Verification items for the finished model (mm, model axes). Face numbers are marked on the shaded views. A direction names the side the tool comes from. Give positions to 0.01 mm unless a question says otherwise; leave off trailing zeros. Loops run counter-clockwise (first coordinate to the right, second up) from the corner with the lowest first, then second, coordinate; pieces in that order, holes last. Notation, with made-up numbers: M -26,-5.75 L 27,-5.75 A22 ccw 27,4.25 Z; hole C 22,46 d5. An arc over 180 degrees is marked long. Put each result on its own line as item: value. Start each with the question number.
from build123d import *

# Parameters (mm, degrees)
F1_DEPTH = 24.85502


# Not quite as in the source:
# - ends of sketch curves that miss each other by under 0.0002 mm in the source are joined


with BuildPart() as f1:
    # F0 (on Top) → F1 (new body)
    with BuildSketch(Plane.XY):
        with BuildLine():
            Line((31.75, -31.7133048595), (44.45, -31.7133048595))
            ThreePointArc((44.45, -31.7133048595), (42.0664322772, -17.3530202013), (35.171359934, -4.5328350256))
            ThreePointArc((35.171359934, -4.5328350256), (33.2360090694, -2.1977123508), (31.1459274206, 0))
            Line((31.1459274206, 0), (1.526038953, 0))
            ThreePointArc((1.526038953, 0), (22.9838447258, -9.8088445461), (31.75, -31.7133048595))
        make_face()
        with BuildLine():
            Line((44.45, -40.8569961303), (44.45, -31.7133048595))
            ThreePointArc((44.45, -31.7133048595), (44.2101126583, -36.3250766164), (43.4930398768, -40.8870708405))
            ThreePointArc((43.4930398768, -40.8870708405), (43.9712837047, -40.8645166634), (44.45, -40.8569961303))
        make_face()
        with BuildLine():
            ThreePointArc((43.4930398768, -40.8870708405), (44.2101126583, -36.3250766164), (44.45, -31.7133048595))
            Line((44.45, -31.7133048595), (31.75, -31.7133048595))
            ThreePointArc((31.75, -31.7133048595), (22.4506403027, -54.1639451622), (0, -63.4633048595))
            Line((0, -63.4633048595), (31.1085197333, -63.4633048595))
            ThreePointArc((31.1085197333, -63.4633048595), (31.0883782789, -48.7672850184), (43.4930398768, -40.8870708405))
        make_face()
        with BuildLine():
            ThreePointArc((35.171359934, -4.5328350256), (42.0664322772, -17.3530202013), (44.45, -31.7133048595))
            Line((44.45, -31.7133048595), (44.45, -4.5328350256))
            Line((44.45, -4.5328350256), (35.171359934, -4.5328350256))
        make_face()
        with BuildLine():
            Line((44.45, -4.5328350256), (44.45, -31.7133048595))
            Line((44.45, -31.7133048595), (44.45, -40.8569961303))
            ThreePointArc((44.45, -40.8569961303), (52.1958071052, -42.9722076639), (57.7914802832, -48.730687431))
            ThreePointArc((57.7914802832, -48.730687431), (63.7666518684, -28.0228983697), (84.4744408875, -33.9980701011))
            ThreePointArc((84.4744408875, -33.9980701011), (90.4496122897, -13.290280973), (111.1574013682, -19.2654525473))
            ThreePointArc((111.1574013682, -19.2654525473), (109.2588815999, -11.8991437909), (111.1574013333, -4.5328350256))
            Line((111.1574013333, -4.5328350256), (44.45, -4.5328350256))
        make_face()
        with BuildLine():
            ThreePointArc((44.45, -40.8569961303), (43.9712837047, -40.8645166634), (43.4930398768, -40.8870708405))
            ThreePointArc((43.4930398768, -40.8870708405), (38.9713966864, -53.0916289358), (31.1085197333, -63.4633048595))
            Line((31.1085197333, -63.4633048595), (44.45, -56.0969961303))
            Line((44.45, -56.0969961303), (44.45, -40.8569961303))
        make_face()
        with BuildLine():
            ThreePointArc((31.1085197333, -63.4633048595), (38.9713966864, -53.0916289358), (43.4930398768, -40.8870708405))
            ThreePointArc((43.4930398768, -40.8870708405), (31.0883782789, -48.7672850184), (31.1085197333, -63.4633048595))
        make_face()
        with BuildLine():
            ThreePointArc((57.7914802832, -48.730687431), (52.1958071052, -42.9722076639), (44.45, -40.8569961303))
            Line((44.45, -40.8569961303), (44.45, -56.0969961303))
            Line((44.45, -56.0969961303), (57.7914802667, -48.7306874011))
        make_face()
        with BuildLine():
            Line((1.526038953, 0), (31.1459274206, 0))
            ThreePointArc((31.1459274206, 0), (0, 12.7366951405), (-31.1459274206, 0))
            Line((-31.1459274206, 0), (-1.526038953, 0))
            ThreePointArc((-1.526038953, 0), (0, 0.0366951405), (1.526038953, 0))
        make_face()
        with BuildLine():
            ThreePointArc((-31.1085197333, -63.4633048595), (0, -76.1633048595), (31.1085197333, -63.4633048595))
            Line((31.1085197333, -63.4633048595), (0, -63.4633048595))
            Line((0, -63.4633048595), (-31.1085197333, -63.4633048595))
        make_face()
        with BuildLine():
            Line((-31.1085197333, -63.4633048595), (0, -63.4633048595))
            ThreePointArc((0, -63.4633048595), (-22.4506403027, -54.1639451622), (-31.75, -31.7133048595))
            Line((-31.75, -31.7133048595), (-44.45, -31.7133048595))
            ThreePointArc((-44.45, -31.7133048595), (-44.2101126583, -36.3250766164), (-43.4930398768, -40.8870708405))
            ThreePointArc((-43.4930398768, -40.8870708405), (-33.340506936, -45.6645101437), (-29.21, -56.0969961303))
            ThreePointArc((-29.21, -56.0969961303), (-29.6922603481, -59.9005103432), (-31.1085197333, -63.4633048595))
        make_face()
        with BuildLine():
            Line((137.8403618666, -4.5328350256), (111.1574013333, -4.5328350256))
            ThreePointArc((111.1574013333, -4.5328350256), (109.2588815999, -11.8991437909), (111.1574013682, -19.2654525473))
            Line((111.1574013333, -19.2654524841), (137.8403618666, -4.5328350256))
        make_face()
        with BuildLine():
            ThreePointArc((84.4744408875, -33.9980701011), (63.7666518684, -28.0228983697), (57.7914802832, -48.730687431))
            Line((57.7914802832, -48.730687431), (84.4744408875, -33.9980701011))
        make_face()
        with BuildLine():
            Line((84.4744408, -33.9980699426), (57.7914802667, -48.7306874011))
            ThreePointArc((57.7914802667, -48.7306874011), (74.9364747628, -56.1221183194), (86.3729605333, -41.3643786718))
            ThreePointArc((86.3729605333, -41.3643786718), (85.8907002078, -37.5608645466), (84.4744408, -33.9980699426))
        make_face()
        with BuildLine():
            Line((-1.526038953, 0), (-31.1459274206, 0))
            ThreePointArc((-31.1459274206, 0), (-33.2360090694, -2.1977123508), (-35.171359934, -4.5328350256))
            ThreePointArc((-35.171359934, -4.5328350256), (-42.0664322772, -17.3530202013), (-44.45, -31.7133048595))
            Line((-44.45, -31.7133048595), (-31.75, -31.7133048595))
            ThreePointArc((-31.75, -31.7133048595), (-22.9838447258, -9.8088445461), (-1.526038953, 0))
        make_face()
        with BuildLine():
            Line((-44.45, -56.0969961303), (-31.1085197333, -63.4633048595))
            ThreePointArc((-31.1085197333, -63.4633048595), (-38.9713966864, -53.0916289358), (-43.4930398768, -40.8870708405))
            ThreePointArc((-43.4930398768, -40.8870708405), (-43.9712837047, -40.8645166634), (-44.45, -40.8569961303))
            Line((-44.45, -40.8569961303), (-44.45, -56.0969961303))
        make_face()
        with BuildLine():
            ThreePointArc((-43.4930398768, -40.8870708405), (-38.9713966864, -53.0916289358), (-31.1085197333, -63.4633048595))
            ThreePointArc((-31.1085197333, -63.4633048595), (-29.6922603481, -59.9005103432), (-29.21, -56.0969961303))
            ThreePointArc((-29.21, -56.0969961303), (-33.340506936, -45.6645101437), (-43.4930398768, -40.8870708405))
        make_face()
        with BuildLine():
            ThreePointArc((113.0559210666, -26.6317612133), (112.5736607275, -22.8282470353), (111.1574013682, -19.2654525473))
            Line((111.1574013682, -19.2654525473), (84.4744408, -33.9980699426))
            ThreePointArc((84.4744408, -33.9980699426), (101.6194353672, -41.3895008426), (113.0559210666, -26.6317612133))
        make_face()
        with BuildLine():
            Line((84.4744408, -33.9980699426), (111.1574013333, -19.2654524841))
            ThreePointArc((111.1574013333, -19.2654524841), (90.4496122897, -13.290280973), (84.4744408, -33.9980699426))
        make_face()
        with BuildLine():
            Line((137.8403618666, -4.5328350256), (111.1574013333, -19.2654524841))
            ThreePointArc((111.1574013682, -19.2654525473), (128.3023958478, -26.6568833977), (139.7388815999, -11.8991437549))
            ThreePointArc((139.7388815999, -11.8991437549), (139.2566212518, -8.0956295419), (137.8403618666, -4.5328350256))
        make_face()
        with BuildLine():
            ThreePointArc((-44.45, -31.7133048595), (-42.0664322772, -17.3530202013), (-35.171359934, -4.5328350256))
            Line((-35.171359934, -4.5328350256), (-111.1574013333, -4.5328350256))
            ThreePointArc((-111.1574013333, -4.5328350256), (-109.7411419481, -8.0956295419), (-109.2588815999, -11.8991437548))
            ThreePointArc((-109.2588815999, -11.8991437548), (-109.7411419274, -15.7026578875), (-111.1574012531, -19.265452339))
            ThreePointArc((-111.1574012531, -19.265452339), (-94.0124067734, -11.8740215822), (-82.5759210666, -26.6317612133))
            ThreePointArc((-82.5759210666, -26.6317612133), (-83.058181437, -30.4352755127), (-84.4744408863, -33.9980700989))
            ThreePointArc((-84.4744408863, -33.9980700989), (-67.3294464068, -26.6066389977), (-55.8929605333, -41.3643786718))
            ThreePointArc((-55.8929605333, -41.3643786718), (-56.3752208889, -45.1678929135), (-57.7914802953, -48.730687453))
            ThreePointArc((-57.7914802953, -48.730687453), (-52.1958071161, -42.9722076703), (-44.45, -40.8569961303))
            Line((-44.45, -40.8569961303), (-44.45, -31.7133048595))
        make_face()
        with BuildLine():
            ThreePointArc((-44.45, -40.8569961303), (-43.9712837047, -40.8645166634), (-43.4930398768, -40.8870708405))
            ThreePointArc((-43.4930398768, -40.8870708405), (-44.2101126583, -36.3250766164), (-44.45, -31.7133048595))
            Line((-44.45, -31.7133048595), (-44.45, -40.8569961303))
        make_face()
        with BuildLine():
            Line((-57.7914802667, -48.7306874011), (-44.45, -56.0969961303))
            Line((-44.45, -56.0969961303), (-44.45, -40.8569961303))
            ThreePointArc((-44.45, -40.8569961303), (-52.1958071161, -42.9722076703), (-57.7914802953, -48.730687453))
        make_face()
        with BuildLine():
            ThreePointArc((-84.4744408863, -33.9980700989), (-78.4992692104, -54.7058589673), (-57.7914802953, -48.730687453))
            Line((-57.7914802953, -48.730687453), (-84.4744408863, -33.9980700989))
        make_face()
        with BuildLine():
            Line((-84.4744408, -33.9980699426), (-57.7914802667, -48.7306874011))
            ThreePointArc((-57.7914802667, -48.7306874011), (-56.3752208889, -45.1678929135), (-55.8929605333, -41.3643786718))
            ThreePointArc((-55.8929605333, -41.3643786718), (-67.3294464068, -26.6066389977), (-84.4744408, -33.9980699426))
        make_face()
        with BuildLine():
            ThreePointArc((-109.2588815999, -11.8991437548), (-109.7411419481, -8.0956295419), (-111.1574013333, -4.5328350256))
            Line((-111.1574013333, -4.5328350256), (-137.8403618666, -4.5328350256))
            Line((-137.8403618666, -4.5328350256), (-111.1574013333, -19.2654524841))
            ThreePointArc((-111.1574013333, -19.2654524841), (-109.7411419274, -15.7026578875), (-109.2588815999, -11.8991437548))
        make_face()
        with BuildLine():
            ThreePointArc((-111.1574012531, -19.265452339), (-105.1822299466, -39.9732413968), (-84.4744408863, -33.9980700989))
            Line((-84.4744408863, -33.9980700989), (-111.1574012531, -19.265452339))
        make_face()
        with BuildLine():
            Line((-111.1574013333, -19.2654524841), (-84.4744408, -33.9980699426))
            ThreePointArc((-84.4744408, -33.9980699426), (-83.058181437, -30.4352755127), (-82.5759210666, -26.6317612133))
            ThreePointArc((-82.5759210666, -26.6317612133), (-94.0124067734, -11.8740215822), (-111.1574013333, -19.2654524841))
        make_face()
        with BuildLine():
            Line((-111.1574013333, -19.2654524841), (-137.8403618666, -4.5328350256))
            ThreePointArc((-137.8403618666, -4.5328350256), (-131.8651902566, -25.2406240616), (-111.1574013333, -19.2654524841))
        make_face()
    extrude(amount=F1_DEPTH)


solid = f1.part
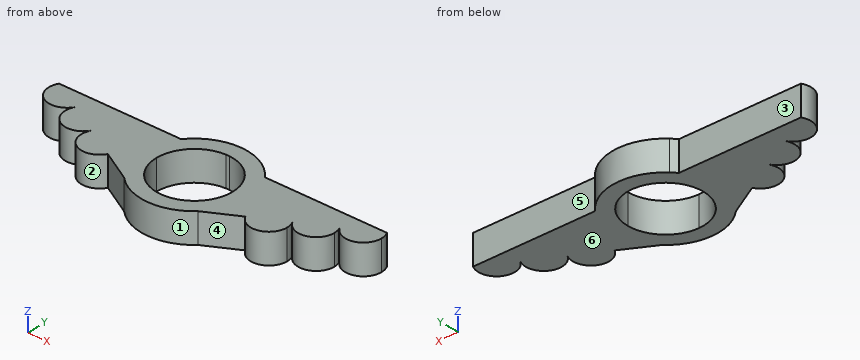
Q1. Set-up check for the marked faces 4, 5 and 6: record each of +Z, -Z, +X, -X, +Y, -Y from which the full face is reachable in a straight line by a thin tool's end or side.
Q2. Cross-section at A-A, the plane z = 3.25. Record the boundary of the cut face in (x, y).
Q3. Go/stop test with flat-tipped pins: pin 1 (7.5 mm diameter, centred on x = 70.5, z = 13, fed in from +Y); pin 2 (1 mm diameter, centred on x = 33, z = 6.5, fed in from +Y); pin 3 (1 mm diameter, centred on y = -48.5, z = 9, fed in from -X). Record where each tip stops, or that it passes through.
Q4. Cross-section at C-C, the plane y = 5. Record the boundary of the cut face in (x, z).
Q5. Scan lines: L1, parallel to X at y = -50, z = 8.5; L2, parallel to X at y = -21.5, z = 3; L3, parallel to X at y = -45, z = 5.25. Record each from-to range of solid material in increasing order.
Q6. Cross-section at B-B, the plane x = -117.5. Record the boundary of the cut face in (y, z).
Q7. Release check for a two-part mould opening along X. For the marked faces 1, 2 and 3 record: pulls with the +X half, pulls with the -X half, needs draft (parallel to the pull), parting line crosses it, or undercut.
Ans:
1. face 4: +Z, -Z, -Y
1. face 5: +Z, -Z, +X, +Y
1. face 6: -Z, +X, -X, +Y, -Y
2. outline: M -137.84,-4.53 A15.24 ccw -111.16,-19.27 A15.24 ccw -84.47,-34 A15.24 ccw -57.79,-48.73 L -31.11,-63.46 A44.45 ccw 31.11,-63.46 L 57.79,-48.73 A15.24 ccw 84.47,-34 A15.24 ccw 111.16,-19.27 A15.24 ccw 137.84,-4.53 L 35.17,-4.53 A44.45 ccw -35.17,-4.53 Z; hole C 0,-31.71 d63.5
3. pin 1: stops at y = -4.53
3. pin 2: stops at y = -1.39
3. pin 3: stops at x = -84.85
4. outline: M -25.06,0 L 25.06,0 L 25.06,24.86 L -25.06,24.86 Z
5. L1: x = -83.69 to -58.58, -55.49 to -25.95, 25.95 to 55.49, 58.58 to 83.69
5. L2: x = -136.33 to -112.66, -112.17 to -30.06, 30.06 to 112.17, 112.66 to 136.33
5. L3: x = -85.93 to -28.84, 28.84 to 85.93
6. outline: M -25.44,0 L -4.53,0 L -4.53,24.86 L -25.44,24.86 Z
7. face 1: parting line crosses it
7. face 2: undercut
7. face 3: needs draft
